```python
from build123d import *

# Parameters (mm, degrees)
F0_R          = 1.75
F1_DEPTH      = 15.875
F3_DEPTH      = 31.75
F4_R          = 3
F5_W          = 5
F5_H          = 35
F6_DEPTH      = 10.001
F6_DEPTH_BACK = 7.5573491861
F7_T1_DEPTH   = 8.7055800262
F7_T3_DEPTH   = 8.75
F7_T5_DEPTH   = 8.75
F7_T7_DEPTH   = 8.7055800262
F8_DEPTH      = 0.3
F9_DEPTH      = 0.3
F10_DEPTH     = 5.3
F11_DEPTH     = 5.3


# Not quite as in the source:
# - a fillet or chamfer that OpenCascade refuses, or shapes differently, is made with other operations: its cross-section is extruded or revolved along the edge and cut away or added


with BuildPart() as f1:
    # F0 (on Right) → F1 (new body, symmetric)
    with BuildSketch(Plane.YZ):
        with BuildLine():
            Line((-5.2303039929, -1.5), (-4.7696960071, -1.5))
            ThreePointArc((-4.7696960071, -1.5), (5, 0), (-4.7696960071, 1.5))
            Line((-4.7696960071, 1.5), (-35, 1.5))
            Line((-35, 1.5), (-42.5, -6))
            Line((-42.5, -6), (-77.5, -6))
            Line((-77.5, -6), (-90.4705627485, 6.9705627485))
            ThreePointArc((-90.4705627485, 6.9705627485), (-93.2989898732, 6.9705627485), (-93.2989898732, 4.1421356237))
            Line((-93.2989898732, 4.1421356237), (-79.1568542495, -10))
            Line((-79.1568542495, -10), (-40.8431457505, -10))
            Line((-40.8431457505, -10), (-32.3431457505, -1.5))
            Line((-32.3431457505, -1.5), (-14.7696960071, -1.5))
            ThreePointArc((-14.7696960071, -1.5), (-10, -5), (-5.2303039929, -1.5))
        make_face()
        Circle(F0_R, mode=Mode.SUBTRACT)
    extrude(amount=F1_DEPTH, both=True)

    # F2 (on face) → F3 (join, through all)
    with BuildSketch(Plane.YZ.offset(15.875)):
        with BuildLine():
            ThreePointArc((-5.2303039929, -1.5), (-7.0419601085, -4.0311288741), (-10, -5))
            Line((-10, -5), (0, -5))
            ThreePointArc((0, -5), (-2.9580398915, -4.0311288741), (-4.7696960071, -1.5))
            Line((-4.7696960071, -1.5), (-5.2303039929, -1.5))
        make_face()
    extrude(amount=-F3_DEPTH)

    # F4
    f4_edges = [f1.edges().sort_by_distance(p)[0] for p in [
        (0, -4.769696, 1.5),
        (0, -14.769696, -1.5),
        (0, -77.5, -6),
        (0, -79.156854, -10),
        (0, -40.843146, -10),
        (0, -32.343146, -1.5),
        (0, -42.5, -6),
        (0, -35, 1.5),
    ]]
    fillet(f4_edges, radius=F4_R)

    # F5 (on Top) → F6 (cut, two sides)
    with BuildSketch(Plane.XY) as f6_sk:
        with Locations((-13.375, -12.5)):
            Rectangle(F5_W, F5_H)
        with Locations((13.375, -12.5)):
            Rectangle(F5_W, F5_H)
    extrude(amount=-F6_DEPTH, mode=Mode.SUBTRACT)
    extrude(f6_sk.sketch, amount=F6_DEPTH_BACK, mode=Mode.SUBTRACT)

    # F7: fillet of radius 1.5 on 4 edges, made by hand

    # F7_s2 → F7_t1 (cut)
    with BuildSketch(Plane.YZ.offset(10.875)):
        with BuildLine():
            ThreePointArc((-31.3668350211, -1.5118453264), (-30.3932598615, -1.0302531824), (-30, -0.0177679895))
            Line((-30, -0.0177679895), (-29.85, -0.0177679895))
            Line((-29.85, -0.0177679895), (-29.85, -1.5))
            Line((-29.85, -1.5), (-30, -1.65))
            ThreePointArc((-30, -1.65), (-31.1005050634, -1.65), (-31.3535185232, -1.66125306))
            Line((-31.3535185232, -1.66125306), (-31.3668350211, -1.5118453264))
        make_face()
    extrude(amount=F7_T1_DEPTH, mode=Mode.SUBTRACT)

    # F7_s4 → F7_t3 (cut)
    with BuildSketch(Plane.YZ.offset(10.875)):
        with BuildLine():
            ThreePointArc((-30, 0), (-30.4393398282, 1.0606601718), (-31.5, 1.5))
            Line((-31.5, 1.5), (-30, 1.5))
            Line((-30, 1.5), (-30, 0))
        make_face()
    extrude(amount=F7_T3_DEPTH, mode=Mode.SUBTRACT)

    # F7_s6 → F7_t5 (cut)
    with BuildSketch(Plane.YZ.offset(-19.625)):
        with BuildLine():
            ThreePointArc((-30, 0), (-30.4393398282, 1.0606601718), (-31.5, 1.5))
            Line((-31.5, 1.5), (-30, 1.5))
            Line((-30, 1.5), (-30, 0))
        make_face()
    extrude(amount=F7_T5_DEPTH, mode=Mode.SUBTRACT)

    # F7_s8 → F7_t7 (cut)
    with BuildSketch(Plane.YZ.offset(-19.5805800262)):
        with BuildLine():
            ThreePointArc((-31.3668350211, -1.5118453264), (-30.3932598615, -1.0302531824), (-30, -0.0177679895))
            Line((-30, -0.0177679895), (-29.85, -0.0177679895))
            Line((-29.85, -0.0177679895), (-29.85, -1.5))
            Line((-29.85, -1.5), (-30, -1.65))
            ThreePointArc((-30, -1.65), (-31.1005050634, -1.65), (-31.3535185232, -1.66125306))
            Line((-31.3535185232, -1.66125306), (-31.3668350211, -1.5118453264))
        make_face()
    extrude(amount=F7_T7_DEPTH, mode=Mode.SUBTRACT)

    # F8 (cut): a face of the model
    f8_faces = [f1.faces().sort_by_distance(p)[0] for p in [
        (10.875, -9.1101781633, -0.6280033564),
    ]]
    extrude(f8_faces, amount=-F8_DEPTH, mode=Mode.SUBTRACT)

    # F9 (cut): a face of the model
    f9_faces = [f1.faces().sort_by_distance(p)[0] for p in [
        (-10.875, -9.1101781633, -0.6280033564),
    ]]
    extrude(f9_faces, amount=-F9_DEPTH, mode=Mode.SUBTRACT)

    # F10 (cut, through all): a face of the model
    f10_faces = [f1.faces().sort_by_distance(p)[0] for p in [
        (15.875, -86.1987808312, -2.0211113015),
    ]]
    extrude(f10_faces, amount=-F10_DEPTH, mode=Mode.SUBTRACT)

    # F11 (cut, through all): a face of the model
    f11_faces = [f1.faces().sort_by_distance(p)[0] for p in [
        (-15.875, -86.1987808312, -2.0211113015),
    ]]
    extrude(f11_faces, amount=-F11_DEPTH, mode=Mode.SUBTRACT)


solid = f1.part
```
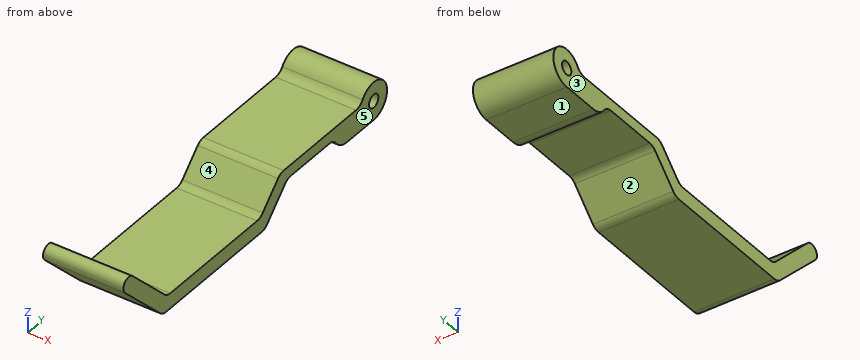
For this review, take the finished solid that the model builds, in its own axes (mm). Face numbers are marked on the shaded views. A direction names the side the tool comes from. Round coordinates to 2 decimals unless told otherwise and drop trailing zeros. Write each loop counter-clockwise with the first axis right and the second up, starting at its lowest first coordinate (ties: lowest second). Pieces come first, ordered by that corner, then holes. Notation, with made-up numbers: (-33, 6) -> (3, 6) arc R13 ccw to (3, 12) -> close; hole circle Ø10 at (8.5, 19). An arc over 180 degrees is marked (long way). One line per question, with ' | ' between items. Start each with the question number.
1) Add section B-B (y = -50). Write out the cut boundary in (x, z) (3 decimals), and give its area (3 significant figures).
2) Add section A-A (x = 2). Write out the cut boundary in (y, z), and give its area (3 significant figures).
3) Wall thickness on line 1 along Z through (x, y) = (5.5, 0); line 2 along Y through (x, z) = (1.5, 0); line 3 along Y through (x, z) = (-5.5, -1): over which ranges is each line inside the solid? List them lowest first.
4) Machinability: for the marked faces 1, 2, 3, 4 and 5, which of the approach directions +Z, -Z, +X, -X, +Y, -Y give a long, thin tool a straight path to every point of the face, cutting with its end or side? Answer none if there is none.
5) Add section C-C (z = -8.25). Write out the cut boundary in (x, y) (3 decimals).
6) For pin 1 Ø12 at (x, y) = (-0.5, -57) entering from +Z; pin 2 Ø7 at (x, y) = (5, -22) entering from -Z; pin 3 Ø10.5 at (x, y) = (-4.5, -17.5) entering from +Z, all flat-tipped, find the tip position at first contact; note any pin that passes through.
Reported:
1) outline: (-10.575, -10) -> (10.575, -10) -> (10.575, -6) -> (-10.575, -6) -> close | area: 84.6 mm²
2) outline: (-93.3, 4.14) -> (-80.04, -9.12) arc R3 ccw to (-77.91, -10) -> (-42.09, -10) arc R3 ccw to (-39.96, -9.12) -> (-33.22, -2.38) arc R3 cw to (-31.1, -1.5) -> (-16.61, -1.5) arc R3 cw to (-14.13, -2.81) arc R5 ccw to (-10, -5) -> (0, -5) arc R5 ccw (long way) to (-4.13, 2.81) arc R3 cw to (-6.61, 1.5) -> (-33.76, 1.5) arc R3 ccw to (-35.88, 0.62) -> (-41.62, -5.12) arc R3 cw to (-43.74, -6) -> (-76.26, -6) arc R3 cw to (-78.38, -5.12) -> (-90.47, 6.97) arc R2 ccw to start; hole circle Ø3.5 at (0, 0) | area: 466 mm²
3) line 1: z = -5 to -1.75, 1.75 to 5 | line 2: y = -89.16 to -83.5, -36.5 to -1.75, 1.75 to 5 | line 3: y = -88.16 to -82.5, -37.5 to -1.44, 1.44 to 4.9
4) face 1: -Z, +X, -X, +Y | face 2: -Z, +X, -X | face 3: +Z, -Z, -X, +Y, -Y | face 4: +Z, +X, -X | face 5: +Z, -Z, +X, +Y, -Y
5) outline: (-10.575, -80.907) -> (10.575, -80.907) -> (10.575, -39.093) -> (-10.575, -39.093) -> close
6) pin 1: stops at z = -6 | pin 2: stops at z = -1.5 | pin 3: stops at z = 1.5
